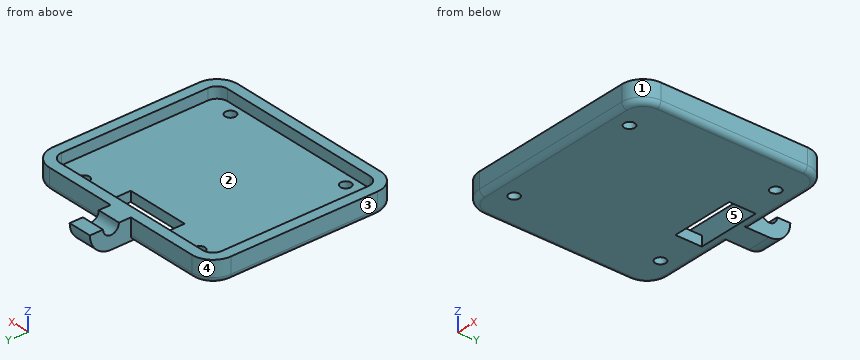
from build123d import *

# Parameters (mm, degrees)
F1_DEPTH      = 4
F3_DEPTH      = 2.1
F5_DEPTH      = 2.25
F5_DEPTH_BACK = 2.25
F6_W          = 12
F6_H          = 5
F6_R          = 1
F7_DEPTH      = 25
F8_R          = 1


with BuildPart() as f1:
    # F0 (on Top) → F1 (new body)
    with BuildSketch(Plane.XY):
        with BuildLine():
            Line((19.85, -13.85), (19.85, 13.85))
            ThreePointArc((19.85, 13.85), (18.678427, 16.678427), (15.85, 17.85))
            Line((15.85, 17.85), (-15.85, 17.85))
            ThreePointArc((-15.85, 17.85), (-18.678427, 16.678427), (-19.85, 13.85))
            Line((-19.85, 13.85), (-19.85, -13.85))
            ThreePointArc((-19.85, -13.85), (-18.678427, -16.678427), (-15.85, -17.85))
            Line((-15.85, -17.85), (15.85, -17.85))
            ThreePointArc((15.85, -17.85), (18.678427, -16.678427), (19.85, -13.85))
        make_face()
    extrude(amount=F1_DEPTH)

    # F2 (on face) → F3 (cut)
    with BuildSketch(Plane.XY.offset(4)):
        with BuildLine():
            ThreePointArc((17.85, 13.85), (17.264214, 15.264214), (15.85, 15.85))
            Line((15.85, 15.85), (-15.85, 15.85))
            ThreePointArc((-15.85, 15.85), (-17.264214, 15.264214), (-17.85, 13.85))
            Line((-17.85, 13.85), (-17.85, -13.85))
            ThreePointArc((-17.85, -13.85), (-17.264214, -15.264214), (-15.85, -15.85))
            Line((-15.85, -15.85), (15.85, -15.85))
            ThreePointArc((15.85, -15.85), (17.264214, -15.264214), (17.85, -13.85))
            Line((17.85, -13.85), (17.85, 13.85))
        make_face()
    extrude(amount=-F3_DEPTH, mode=Mode.SUBTRACT)

    # F4 (on Right) → F5 (join, two sides)
    with BuildSketch(Plane.YZ) as f5_sk:
        with BuildLine():
            Line((17.85, 0), (21.6, 0))
            ThreePointArc((21.6, 0), (24.428427, 1.171573), (25.6, 4))
            Line((25.6, 4), (23.1, 4))
            ThreePointArc((23.1, 4), (21.6, 2.5), (20.1, 4))
            Line((20.1, 4), (17.85, 4))
            Line((17.85, 4), (17.85, 0))
        make_face()
        Polygon((15.85, 0), (17.85, 0), (17.85, 4), (17.6, 4), (15.85, 4), align=None)
    extrude(amount=F5_DEPTH)
    extrude(f5_sk.sketch, amount=-F5_DEPTH_BACK)

    # F6 (on face) → F7 (cut)
    with BuildSketch(Plane.XY.offset(1.9)):
        with Locations((0, 13.35)):
            Rectangle(F6_W, F6_H)
        with Locations((-12.85, 13.85)):
            Circle(F6_R)
        with Locations((12.85, 13.85)):
            Circle(F6_R)
        with Locations((-12.85, -13.85)):
            Circle(F6_R)
        with Locations((12.85, -13.85)):
            Circle(F6_R)
    extrude(amount=-F7_DEPTH, mode=Mode.SUBTRACT)

    # F8
    f8_edges = [f1.edges().sort_by_distance(p)[0] for p in [
        (-19.85, 0, 0),
    ]]
    fillet(f8_edges, radius=F8_R)


solid = f1.part
Work out the finished part from the listing and answer in its coordinate system (mm). Face numbers are marked on the shaded views. A direction names the side the tool comes from. Coordinates: 2 decimals unless noted, no trailing zeros. Write each loop counter-clockwise with the first axis right and the second up, starting at its lowest first coordinate (ties: lowest second). Pieces come first, ordered by that corner, then holes. Notation, with made-up numbers: M 43,-38 L 83,-38 A11 cw 83,-18 Z; hole C -6.5,69.5 d5. An arc over 180 degrees is marked long. Write item = value, one per line.
1. Straight lines are drawn through the part: line 1 (X direction, y = -4, z = 2.2); line 2 (Y direction, x = 5, z = 2.3); line 3 (Y direction, x = 15, z = 1.1). For each, find the intervals that lie inside material, in ascending order. Write a range as from..to.
Solution:
line_1 = -19.85..-17.85, 17.85..19.85
line_2 = -17.85..-15.85, 15.85..17.85
line_3 = -17.85..17.85
2. For the marked faces 4 and 5, determine the directions among +Z, -Z, +X, -X, +Y, -Y from which every point of the face is accessible in a straight line to the end or side of a thin tool.
Solution:
face_4 = +Z, -Z, -X, +Y
face_5 = +Z
3. The part is cut by section D-D (z = 3.05). Determine the outline of the cut face in (x, y).
Solution:
outline = M -19.85,-13.85 A4 ccw -15.85,-17.85 L 15.85,-17.85 A4 ccw 19.85,-13.85 L 19.85,13.85 A4 ccw 15.85,17.85 L 2.25,17.85 L 2.25,20.44 L -2.25,20.44 L -2.25,17.85 L -15.85,17.85 A4 ccw -19.85,13.85 Z; M -2.25,22.76 L 2.25,22.76 L 2.25,25.49 L -2.25,25.49 Z; hole M -17.85,-13.85 A2 ccw -15.85,-15.85 L 15.85,-15.85 A2 ccw 17.85,-13.85 L 17.85,13.85 A2 ccw 15.85,15.85 L -15.85,15.85 A2 ccw -17.85,13.85 Z
4. Determine the mould class of the marked faces 1, 2 and 3 for opening direction Y: released by +Y, released by -Y, zero draft, split by the parting line, or undercut.
Solution:
face_1 = released by -Y
face_2 = undercut
face_3 = zero draft
5. Flat-ended cylindrical pins translate along their axes: pin 1 (2.5 mm diameter, centred on x = 12.85, y = 13.85, fed in from +Z); pin 2 (2 mm diameter, centred on y = 21, z = 2.5, fed in from -X); pin 3 (1 mm diameter, centred on x = 1, z = 2.5, fed in from +Y). Find the tip coordinate at first contact, or state that the pin passes through.
Solution:
pin_1 = 1.9
pin_2 = -2.25
pin_3 = 25.47
6. The part is cut by section B-B (x = -0.5). Determine the outline of the cut face in (y, z).
Solution:
outline = M -17.85,1 A1 ccw -16.85,0 L 10.85,0 L 10.85,1.9 L -15.85,1.9 L -15.85,4 L -17.85,4 Z; M 15.85,0 L 21.6,0 A4 ccw 25.6,4 L 23.1,4 A1.5 cw 20.1,4 L 15.85,4 Z
7. The part is cut by section C-C (y = -7.5). Determine the outline of the cut face in (x, z).
Solution:
outline = M -19.85,1 A1 ccw -18.85,0 L 18.85,0 A1 ccw 19.85,1 L 19.85,4 L 17.85,4 L 17.85,1.9 L -17.85,1.9 L -17.85,4 L -19.85,4 Z
8. The part is cut by section A-A (x = -12.85). Determine the outline of the cut face in (y, z), then the cut area to 3 significant figures.
Solution:
outline = M -17.85,1 A1 ccw -16.85,0 L -14.85,0 L -14.85,1.9 L -15.85,1.9 L -15.85,4 L -17.85,4 Z; M -12.85,0 L 12.85,0 L 12.85,1.9 L -12.85,1.9 Z; M 14.85,0 L 16.85,0 A1 ccw 17.85,1 L 17.85,4 L 15.85,4 L 15.85,1.9 L 14.85,1.9 Z
area = 68.2 mm2
